Drawing for the job (mm, zero at the part's lowest x, y, z). A direction names the side the tool comes from. Give positions to 0.01 mm unless a question says otherwise; leave off trailing zeros. Order: outer loops, then holes, each group sorted by start corner. A loop starts at its lowest first (then second) coordinate and runs counter-clockwise, first axis right, second up. Notation, with made-up numbers: (88, 17.5) -> (135, 17.5) arc R31 cw to (135, 41.5) -> close; hole circle Ø9 at (-6, -34). An arc over 180 degrees is marked (long way). One line per item, written item: value. Start each with the question number.
(1) Probe line 1 (Y direction, x = 15, z = 3.25); line 2 (Y direction, x = 15, z = 1.6); line 3 (Z direction, x = 22.5, y = 27). List the from-to ranges inside material, lowest first.
(2) Saw through at A-A on x = 15. Give the cut face in (y, z).
(3) Saw through at C-C on y = 15. Give the cut face in (x, z).
(4) Saw through at B-B on z = 1.4. Count the separate pieces of the cut face and the enclosed holes in it, plus the area to 3 significant figures.
(5) Saw through at D-D on x = 19.5. Give the cut face in (y, z).
(6) Two-plate mould, pull along Y, no slides. Class the marked faces 1, 2, 3 and 4: +Y half, -Y half, draft (parallel to the pull), parting line (faces both ways), or undercut.
(7) Pin check, flat tips, straight feed: pin 1 (7 mm diameter, centred on x = 15, y = 25, fed in from +Z); pin 2 (1.5 mm diameter, centred on x = 21, z = 2.5, fed in from -Y). Stop position of each tip, or through.
(8) Which spindle directions (+Z, -Z, +X, -X, +Y, -Y) get a long thin tool onto all of the face, cutting with end or side? Do the marked faces 5 and 6. Say none if no direction does.
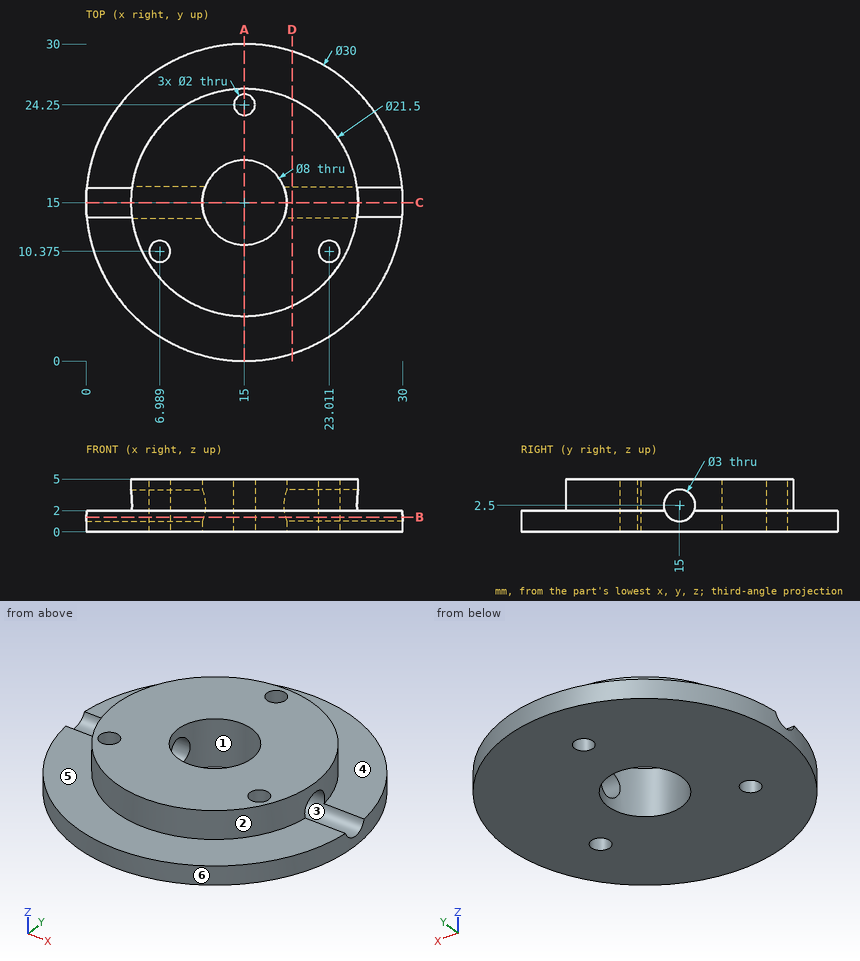
Results below:
1. line 1: y = 4.25 to 11, 19 to 23.25, 25.25 to 25.75
1. line 2: y = 0 to 11, 19 to 23.25, 25.25 to 30
1. line 3: z = 0 to 2
2. outline: (0, 0) -> (11, 0) -> (11, 5) -> (4.25, 5) -> (4.25, 2) -> (0, 2) -> close; (19, 0) -> (23.25, 0) -> (23.25, 5) -> (19, 5) -> close; (25.25, 0) -> (30, 0) -> (30, 2) -> (25.75, 2) -> (25.75, 5) -> (25.25, 5) -> close
3. outline: (0, 0) -> (11, 0) -> (11, 1) -> (0, 1) -> close; (4.25, 4) -> (11, 4) -> (11, 5) -> (4.25, 5) -> close; (19, 0) -> (30, 0) -> (30, 1) -> (19, 1) -> close; (19, 4) -> (25.75, 4) -> (25.75, 5) -> (19, 5) -> close
4. separate pieces: 2
4. enclosed holes: 3
4. area: 602 mm²
5. outline: (0.69, 0) -> (29.31, 0) -> (29.31, 2) -> (24.76, 2) -> (24.76, 5) -> (5.24, 5) -> (5.24, 2) -> (0.69, 2) -> close; hole circle Ø3 at (15, 2.5)
6. face 1: undercut
6. face 2: parting line
6. face 3: undercut
6. face 4: draft
7. pin 1: stops at z = 5
7. pin 2: stops at y = 1.02
8. face 5: +Z, -Y
8. face 6: +Z, -Z
